Design review of the part built by this model. Coordinates are the model's own, in mm. A direction names the side the tool comes from. Coordinates: 2 decimals unless noted, no trailing zeros. Write each loop counter-clockwise with the first axis right and the second up, starting at its lowest first coordinate (ties: lowest second). Pieces come first, ordered by that corner, then holes. Notation, with made-up numbers: (-7.75, -11) -> (18.25, -11) arc R8 cw to (18.25, 4) -> close; hole circle Ø10 at (38, 9.5). An arc over 180 degrees is marked (long way). Write item = value, one per line. Start each with the question number.
Autodesk Inventor part; units mm, degrees
ref_plane "YZ Plane" through (0, 0, 0) normal (1, 0, 0) x (0, 1, 0)
ref_plane "XZ Plane" through (0, 0, 0) normal (0, 1, 0) x (-1, 0, 0)
ref_plane "XY Plane" through (0, 0, 0) normal (0, 0, 1) x (1, 0, 0)
sketch "Sketch1" plane through (0, 0, 0) normal (0, 1, 0) x (-1, 0, 0)
  line L0 (-11.8108, -30.2381) -> (15.1767, -30.2381)
  line L1 (15.1767, -30.2381) -> (15.1767, 5.9569)
  line L2 (15.1767, 5.9569) -> (-11.8108, 5.9569)
  line L3 (-11.8108, 5.9569) -> (-11.8108, -30.2381)
  line L4 (-11.8108, -30.2381) -> (-14.9858, -30.2381)
  line L5 (-14.9858, -30.2381) -> (-14.9858, -17.5381)
  line L6 (-14.9858, -17.5381) -> (-11.8108, -17.5381)
  line L7 (-11.8108, -17.5381) -> (-11.8108, -30.2381)
  line L8 (-11.8108, -8.6481) -> (-14.9858, -8.6481)
  line L9 (-14.9858, -8.6481) -> (-14.9858, 4.0519)
  line L10 (-14.9858, 4.0519) -> (-11.8108, 4.0519)
  line L11 (-11.8108, 4.0519) -> (-11.8108, -8.6481)
  line L12 (-14.9858, -30.2381) -> (-2.2858, -30.2381)
  line L13 (-2.2858, -30.2381) -> (-2.2858, -33.4131)
  line L14 (-2.2858, -33.4131) -> (-14.9858, -33.4131)
  line L15 (-14.9858, -33.4131) -> (-14.9858, -30.2381)
  line L16 (15.1767, -30.2381) -> (6.6042, -30.2381)
  line L17 (6.6042, -30.2381) -> (6.6042, -33.4131)
  line L18 (6.6042, -33.4131) -> (15.1767, -33.4131)
  line L19 (15.1767, -33.4131) -> (15.1767, -30.2381)
  point P0 (0, 0)
  dimension "d0" = 26.9875
  dimension "d1" = 36.195
  dimension "d5" = 3.175
  dimension "d6" = 12.7
  dimension "d7" = 8.89
  dimension "d8" = 12.7
  dimension "d10" = 12.7
  dimension "d11" = 8.89
extrude "Extrusion1" add sketch "Sketch1" along normal blind 3.175
mirror "Mirror1" about plane through (-15.1767, 0, 5.9569) normal (0, 0, 1) of "Extrusion1"
mirror "Mirror2" about plane through (-15.1767, 0, -33.4131) normal (-1, 0, 0) of "Extrusion1", "Mirror1"
sketch "Sketch2" plane through (0, 3.175, 0) normal (0, 1, 0) x (1, 0, 0)
  line L0 (-1.9052, 2.8061) -> (-22.4792, 2.8061)
  line L1 (-22.4792, 2.8061) -> (-22.4792, -17.7679)
  line L2 (-22.4792, -17.7679) -> (-1.9052, -17.7679)
  line L3 (-1.9052, -17.7679) -> (-1.9052, 2.8061)
  line L4 (14.9858, -7.8619) -> (14.9858, -20.5619)
  line L5 (-45.3392, -7.8619) -> (-45.3392, -20.5619)
  line L6 (-23.7492, -45.3269) -> (-6.6042, -45.3269)
  line L7 (-6.6042, 33.4131) -> (-23.7492, 33.4131)
  line L8 (-22.4792, 26.4281) -> (-8.2552, 26.4281)
  line L9 (-8.2552, 26.4281) -> (-8.2552, 33.4131)
  line L10 (-8.2552, 33.4131) -> (-22.4792, 33.4131)
  line L11 (-22.4792, 33.4131) -> (-22.4792, 26.4281)
  point P0 (0, 0)
  dimension "d14" = 20.574
  dimension "d15" = 16.891
  dimension "d16" = 22.86
  dimension "d17" = 27.559
  dimension "d18" = 20.574
  dimension "d19" = 14.224
  dimension "d20" = 6.985
extrude "Extrusion2" cut sketch "Sketch2" against normal blind 3.175
(1) For pin 1 Ø12 at (x, z) = (-37.5, -25) entering from -Y; pin 2 Ø1.6 at (x, y) = (-18.5, 1) entering from -Z; pin 3 Ø12 at (x, z) = (-9.5, 10.5) entering from -Y; pin 4 Ø1 at (x, y) = (0, 1.5) entering from -Z, all flat-tipped, find the tip position at first contact; note any pin that passes through.
(2) Take a section at A-A, the plane z = -28. State the section outline as (x, y) points (3 decimals), then the cut area to 3 significant figures.
(3) For line 1 (Z direction, x = -43, y = 0.5); line 2 (Z direction, x = -18, y = 3); line 3 (X direction, y = 1.9, z = 11), list the stretches that pass through material, from the lowest coordinate up.
(4) For faces 4 (the face through (13, 2, -8.648)), 5 (the face through (-32.639, 2, -32)), 6 (the face through (-1.905, 2, 8)), 7 (the face through (-44, 2, 29.452)), list the 3-axis set-ups (+Z, -Z, +X, -X, +Y, -Y) from which the entire face can be reached by the end or side of a thin tool; tool diameter is ignored.
(5) Take a section at B-B, the plane x = -28.5. State the section outline as (y, z) points (3 decimals).
(6) Mouldability with a two-part tool opening along Z and no side actions: class faces 1 (the face through (-15, 2, 45.327)), 2 (the face through (-28, 0, 7)), 3 (the face through (13, 2, 4.052)) as pulls with the +Z half, pulls with the -Z half, needs draft (parallel to the pull), parting line crosses it, or undercut.
Report:
q1.pin_1 = 0
q1.pin_2 = -26.43
q1.pin_3 = through
q1.pin_4 = -30.24
q2.outline = (-45.339, 0) -> (-22.479, 0) -> (-22.479, 3.175) -> (-45.339, 3.175) -> close; (-8.255, 0) -> (14.986, 0) -> (14.986, 3.175) -> (-8.255, 3.175) -> close
q2.area = 146 mm2
q3.line_1 = -33.41 to -17.54, -8.65 to 4.05, 7.86 to 20.56, 29.45 to 45.33
q3.line_2 = -26.43 to -2.81, 17.77 to 45.33
q3.line_3 = -45.34 to -22.48, -1.91 to 14.99
q4.face_4 = +X, +Y, -Y
q4.face_5 = -Z, +Y, -Y
q4.face_6 = +Y, -Y
q4.face_7 = -X, +Y, -Y
q5.outline = (0, -30.238) -> (3.175, -30.238) -> (3.175, 42.152) -> (0, 42.152) -> close
q6.face_1 = pulls with the +Z half
q6.face_2 = needs draft
q6.face_3 = undercut
